from build123d import *

# Parameters (mm, degrees)
F0_W     = 6
F0_H     = 62
F0_W_2   = 38
F1_DEPTH = 1
F2_DEPTH = 10
F3_R     = 5


# Not quite as in the source:
# - a feature names something its author has since deleted; it is built from what else it names


with BuildPart() as f1:
    # F0 (on Top) → F1 (new body)
    with BuildSketch(Plane.XY):
        with Locations((-12.5, 19)):
            Rectangle(F0_W, F0_H)
        with Locations((9.5, 19)):
            Rectangle(F0_W_2, F0_H)
        with BuildLine():
            ThreePointArc((9.5, 15.8775010008), (10.0985618966, 14.4432029131), (10.9121369044, 13.1189736826))
            Line((10.9121369044, 13.1189736826), (10.9121369044, 5.8810263174))
            ThreePointArc((10.9121369044, 5.8810263174), (10.0985618966, 4.5567970869), (9.5, 3.1224989992))
            ThreePointArc((9.5, 3.1224989992), (8.9014381034, 4.5567970869), (8.0878630956, 5.8810263174))
            Line((8.0878630956, 5.8810263174), (8.0878630956, 13.1189736826))
            ThreePointArc((8.0878630956, 13.1189736826), (8.9014381034, 14.4432029131), (9.5, 15.8775010008))
        make_face(mode=Mode.SUBTRACT)
        with BuildLine():
            Line((8.0878630956, 24.8810263174), (8.0878630956, 32.1189736826))
            ThreePointArc((8.0878630956, 32.1189736826), (8.9014381034, 33.4432029131), (9.5, 34.8775010008))
            ThreePointArc((9.5, 34.8775010008), (10.0985618966, 33.4432029131), (10.9121369044, 32.1189736826))
            Line((10.9121369044, 32.1189736826), (10.9121369044, 24.8810263174))
            ThreePointArc((10.9121369044, 24.8810263174), (10.0985618966, 23.5567970869), (9.5, 22.1224989992))
            ThreePointArc((9.5, 22.1224989992), (8.9014381034, 23.5567970869), (8.0878630956, 24.8810263174))
        make_face(mode=Mode.SUBTRACT)
    extrude(amount=F1_DEPTH)

    # F0 (on Top) → F2 (join)
    with BuildSketch(Plane.XY):
        with BuildLine():
            ThreePointArc((9.5, 34.8775010008), (8.9014381034, 33.4432029131), (8.0878630956, 32.1189736826))
            Line((8.0878630956, 32.1189736826), (8.0878630956, 24.8810263174))
            ThreePointArc((8.0878630956, 24.8810263174), (8.9014381034, 23.5567970869), (9.5, 22.1224989992))
            ThreePointArc((9.5, 22.1224989992), (10.0985618966, 23.5567970869), (10.9121369044, 24.8810263174))
            Line((10.9121369044, 24.8810263174), (10.9121369044, 32.1189736826))
            ThreePointArc((10.9121369044, 32.1189736826), (10.0985618966, 33.4432029131), (9.5, 34.8775010008))
        make_face()
        with BuildLine():
            Line((10.9121369044, 5.8810263174), (10.9121369044, 13.1189736826))
            ThreePointArc((10.9121369044, 13.1189736826), (10.0985618966, 14.4432029131), (9.5, 15.8775010008))
            ThreePointArc((9.5, 15.8775010008), (8.9014381034, 14.4432029131), (8.0878630956, 13.1189736826))
            Line((8.0878630956, 13.1189736826), (8.0878630956, 5.8810263174))
            ThreePointArc((8.0878630956, 5.8810263174), (8.9014381034, 4.5567970869), (9.5, 3.1224989992))
            ThreePointArc((9.5, 3.1224989992), (10.0985618966, 4.5567970869), (10.9121369044, 5.8810263174))
        make_face()
    extrude(amount=F2_DEPTH)

    # F3
    f3_edges = [f1.edges().sort_by_distance(p)[0] for p in [
        (-15.5, 50, 0.5),
        (28.5, 50, 0.5),
        (28.5, -12, 0.5),
        (-15.5, -12, 0.5),
    ]]
    fillet(f3_edges, radius=F3_R)


solid = f1.part
Build history of the part. All positions in model axes, mm. A direction names the side the tool comes from. Give positions to 0.01 mm unless a question says otherwise; leave off trailing zeros. Loops run counter-clockwise (first coordinate to the right, second up) from the corner with the lowest first, then second, coordinate; pieces in that order, holes last. Notation, with made-up numbers: (17, 42) -> (23, 42) arc R19 cw to (23, 61) -> close; hole circle Ø5 at (-34, 29). An arc over 180 degrees is marked (long way). Answer in a Markdown table with one row per item.
Item 1: Flat gauge pins, fed straight in: P1, Ø3.5, axis at y = 29, z = 7, coming from the +X side; P2, Ø6, axis at y = 27, z = 5, coming from the -X side; P3, Ø6, axis at x = 18, y = 19, coming from the +Z side. Where does each tip first touch, or does it go through?
Findings below:
| item | result |
|---|---|
| P1 | stops at x = 10.91 |
| P2 | stops at x = 8.09 |
| P3 | stops at z = 1 |
Item 2: Mould opens along Y. For faces 5 (the cylindrical face through (27, 48.57, 0.51)), 6 (the flat face through (9, 29, 10)), 7 (the cylindrical face through (8.89, 23.58, 5.44)) say: pulls with the +Y half, pulls with the -Y half, needs draft (parallel to the pull), parting line crosses it, or undercut.
Findings below:
| item | result |
|---|---|
| face 5 | pulls with the +Y half |
| face 6 | needs draft |
| face 7 | undercut |
Item 3: Slice it at B-B on y = 24. Write the cut outline in (x, z).
Findings below:
| item | result |
|---|---|
| outline | (-15.5, 0) -> (28.5, 0) -> (28.5, 1) -> (10.34, 1) -> (10.34, 10) -> (8.66, 10) -> (8.66, 1) -> (-15.5, 1) -> close |
Item 4: Probe line 1 along X through (y, z) = (7, 1.75); line 2 along Z through (x, y) = (22, 47); line 3 along Y through (x, z) = (10.5, 8.25). List the from-to ranges inside material, lowest first. Write a range as [from, to].
Findings below:
| item | result |
|---|---|
| line 1 | x = [8.09, 10.91] |
| line 2 | z = [0, 1] |
| line 3 | y = [5.27, 13.73], [24.27, 32.73] |
Item 5: Slice it at D-D on y = 37. Write the cut outline in (x, z).
Findings below:
| item | result |
|---|---|
| outline | (-15.5, 0) -> (28.5, 0) -> (28.5, 1) -> (-15.5, 1) -> close |
Item 6: Tool access for faces 1 (the cylindrical face through (10.11, 14.42, 5.44)), 2 (the flat face through (8.088, 29, 5)), 3 (the cylindrical face through (10.11, 33.42, 5.44)), 4 (the cylindrical face through (8.91, 33.46, 5.44)): list every direction of +Z, -Z, +X, -X, +Y, -Y with a clear straight run to the whole face (end or side of a thin tool).
Findings below:
| item | result |
|---|---|
| face 1 | +Z, +X |
| face 2 | +Z, -X, +Y, -Y |
| face 3 | +Z, +X, +Y |
| face 4 | +Z, -X, +Y |
Item 7: Slice it at A-A on z = 4.75. Write the cut outline in (x, y), plus the area to 3 significant figures.
Findings below:
| item | result |
|---|---|
| outline | (8.09, 5.88) arc R10 cw to (9.5, 3.12) arc R10 cw to (10.91, 5.88) -> (10.91, 13.12) arc R10 cw to (9.5, 15.88) arc R10 cw to (8.09, 13.12) -> close; (8.09, 24.88) arc R10 cw to (9.5, 22.12) arc R10 cw to (10.91, 24.88) -> (10.91, 32.12) arc R10 cw to (9.5, 34.88) arc R10 cw to (8.09, 32.12) -> close |
| area | 54.5 mm² |
Item 8: Slice it at C-C on x = 19. Write the cut outline in (y, z), plus the area to 3 significant figures.
Findings below:
| item | result |
|---|---|
| outline | (-12, 0) -> (50, 0) -> (50, 1) -> (-12, 1) -> close |
| area | 62.0 mm² |
